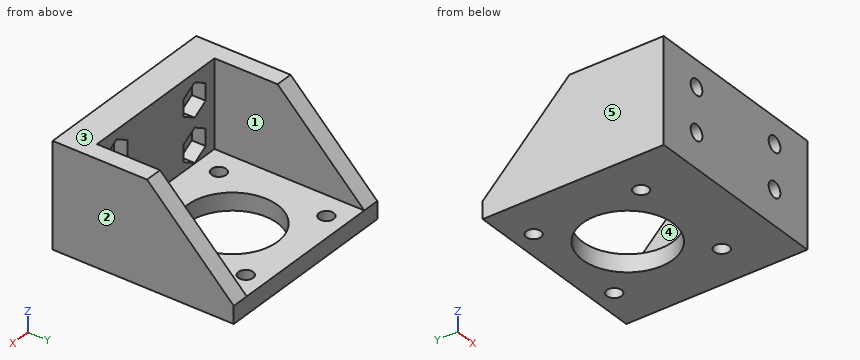
```python
from build123d import *

# Parameters (mm, degrees)
F0_R     = 2.125
F0_R_2   = 13
F1_DEPTH = 5
F3_DEPTH = 25
F4_W     = 55.2
F4_H     = 30
F4_R     = 2.25
F5_DEPTH = 5
F6_W     = 45.2
F6_H     = 25
F7_DEPTH = 4
F8_SIZE  = 25


with BuildPart() as f1:
    # F0 (on Top) → F1 (new body)
    with BuildSketch(Plane.XY):
        Polygon((27.6, -21.1), (27.6, 21.1), (-27.6, 21.1), (-27.6, -21.1), (-27.6, -31.1), (0, -31.1), (27.6, -31.1), align=None)
        with Locations((-15.5, -15.5)):
            Circle(F0_R, mode=Mode.SUBTRACT)
        with Locations((15.5, -15.5)):
            Circle(F0_R, mode=Mode.SUBTRACT)
        with Locations((-15.5, 15.5)):
            Circle(F0_R, mode=Mode.SUBTRACT)
        Circle(F0_R_2, mode=Mode.SUBTRACT)
        with Locations((15.5, 15.5)):
            Circle(F0_R, mode=Mode.SUBTRACT)
    extrude(amount=F1_DEPTH)

    # F2 (on face) → F3 (join)
    with BuildSketch(Plane.XY.offset(5)):
        Polygon((-22.6, -21.1), (-22.6, 21.1), (-27.6, 21.1), (-27.6, -21.1), (-27.6, -31.1), (-22.6, -31.1), align=None)
        Polygon((27.6, 21.1), (22.6, 21.1), (22.6, -21.1), (22.6, -31.1), (27.6, -31.1), (27.6, -21.1), align=None)
    extrude(amount=F3_DEPTH)

    # F4 (on face) → F5 (join)
    with BuildSketch(Plane.XZ.offset(31.1)):
        with Locations((0, 15)):
            Rectangle(F4_W, F4_H)
        with Locations((-15, 10)):
            Circle(F4_R, mode=Mode.SUBTRACT)
        with Locations((15, 10)):
            Circle(F4_R, mode=Mode.SUBTRACT)
        with Locations((-15, 22.5)):
            Circle(F4_R, mode=Mode.SUBTRACT)
        with Locations((15, 22.5)):
            Circle(F4_R, mode=Mode.SUBTRACT)
    extrude(amount=-F5_DEPTH)

    # F6 (on face) → F7 (join)
    with BuildSketch(Plane(origin=(0, -26.1, 0), x_dir=(-1, 0, 0), z_dir=(0, 1, 0))):
        with Locations((0, 17.5)):
            Rectangle(F6_W, F6_H)
        Polygon((-15, 14.87861), (-10.775, 12.439305), (-10.775, 7.560695), (-15, 5.12139), (-19.225, 7.560695), (-19.225, 12.439305), align=None, mode=Mode.SUBTRACT)
        Polygon((10.775, 7.560695), (10.775, 12.439305), (15, 14.87861), (19.225, 12.439305), (19.225, 7.560695), (15, 5.12139), align=None, mode=Mode.SUBTRACT)
        Polygon((-15, 27.37861), (-10.775, 24.939305), (-10.775, 20.060695), (-15, 17.62139), (-19.225, 20.060695), (-19.225, 24.939305), align=None, mode=Mode.SUBTRACT)
        Polygon((10.775, 24.939305), (15, 27.37861), (19.225, 24.939305), (19.225, 20.060695), (15, 17.62139), (10.775, 20.060695), align=None, mode=Mode.SUBTRACT)
    extrude(amount=F7_DEPTH)

    # F8
    f8_edges = [f1.edges().sort_by_distance(p)[0] for p in [
        (-25.1, 21.1, 30),
        (25.1, 21.1, 30),
    ]]
    chamfer(f8_edges, length=F8_SIZE)


solid = f1.part
```
Part model, mm, in its own coordinate system. Face numbers are marked on the shaded views. A direction names the side the tool comes from. Coordinates: 2 decimals unless noted, no trailing zeros. Write each loop counter-clockwise with the first axis right and the second up, starting at its lowest first coordinate (ties: lowest second). Pieces come first, ordered by that corner, then holes.
Item 1: Which spindle directions (+Z, -Z, +X, -X, +Y, -Y) get a long thin tool onto all of the face, cutting with end or side? Do the marked faces 4 and 5. Say none if no direction does.
Item 2: Slice it at A-A (z = 4). Write the cut outline in (x, y) (3 decimals).
Item 3: Slice it at D-D (y = 15.5). Write the cut outline in (x, z) (3 decimals), and give its area (4 significant figures).
Item 4: Slice it at C-C (z = 9). Write the cut outline in (x, y) (3 decimals).
Item 5: Probe line 1 (Z direction, x = 15, y = -29); line 2 (Y direction, x = -15.5, z = 1.1) (3 decimals); line 3 (X direction, y = 14.5, z = 11.5). List the from-to ranges inside material, lowest first.
Item 6: Mould opens along X. For the marked faces 1, 2 and 3 say: released by +X, released by -X, zero draft, split by the parting line, or undercut.
Item 7: Slice it at B-B (y = -15.5). Write the cut outline in (x, z) (3 decimals), and give its area (4 significant figures).
Item 8: Pin check, flat tips, straight feed: pin 1 (1.5 mm diameter, centred on x = 17, y = -16, fed in from +Z); pin 2 (3.5 mm diameter, centred on x = 15, z = 10, fed in from +Y); pin 3 (4 mm diameter, centred on x = 14.5, z = 21, fed in from +Y); pin 4 (7.5 mm diameter, centred on x = 7, z = 14.5, fed in from +Y). Stop position of each tip, or through.
Results found:
1. face 4: +Z, +Y
1. face 5: +Z, -Z, -X, +Y, -Y
2. outline: (-27.6, -31.1) - (27.6, -31.1) - (27.6, 21.1) - (-27.6, 21.1) - close; hole circle Ø4.25 at (-15.5, -15.5); hole circle Ø4.25 at (-15.5, 15.5); hole circle Ø26 at (0, 0); hole circle Ø4.25 at (15.5, -15.5); hole circle Ø4.25 at (15.5, 15.5)
3. outline: (-27.6, 0) - (-17.625, 0) - (-17.625, 5) - (-22.6, 5) - (-22.6, 10.6) - (-27.6, 10.6) - close; (-13.375, 0) - (13.375, 0) - (13.375, 5) - (-13.375, 5) - close; (17.625, 0) - (27.6, 0) - (27.6, 10.6) - (22.6, 10.6) - (22.6, 5) - (17.625, 5) - close
3. area: 289.5 mm2
4. outline: (-27.6, -31.1) - (-17.016, -31.1) - (-17.016, -26.1) - (-19.225, -26.1) - (-19.225, -22.1) - (-22.6, -22.1) - (-22.6, 17.1) - (-27.6, 17.1) - close; (-12.984, -31.1) - (12.984, -31.1) - (12.984, -26.1) - (10.775, -26.1) - (10.775, -22.1) - (-10.775, -22.1) - (-10.775, -26.1) - (-12.984, -26.1) - close; (17.016, -31.1) - (27.6, -31.1) - (27.6, 17.1) - (22.6, 17.1) - (22.6, -22.1) - (19.225, -22.1) - (19.225, -26.1) - (17.016, -26.1) - close
5. line 1: z = 0 to 7.75, 12.25 to 20.25, 24.75 to 30
5. line 2: y = -31.1 to -17.625, -13.375 to 13.375, 17.625 to 21.1
5. line 3: x = -27.6 to -22.6, 22.6 to 27.6
6. face 1: undercut
6. face 2: released by +X
6. face 3: zero draft
7. outline: (-27.6, 0) - (-17.625, 0) - (-17.625, 5) - (-22.6, 5) - (-22.6, 30) - (-27.6, 30) - close; (-13.375, 0) - (13.375, 0) - (13.375, 5) - (-13.375, 5) - close; (17.625, 0) - (27.6, 0) - (27.6, 30) - (22.6, 30) - (22.6, 5) - (17.625, 5) - close
7. area: 483.5 mm2
8. pin 1: stops at z = 5
8. pin 2: passes through
8. pin 3: stops at y = -26.1
8. pin 4: stops at y = -22.1
